For this review, take the finished solid that the model builds, in its own axes (mm). A direction names the side the tool comes from. Give positions to 0.01 mm unless a question says otherwise; leave off trailing zeros. Write each loop counter-clockwise with the first axis right and the second up, starting at its lowest first coordinate (ties: lowest second). Pieces come first, ordered by that corner, then holes.
1) For P1, Ø3, axis at x = 16, z = 97, coming from the +Y side; P2, Ø3, axis at x = -2.5, y = 36.5, coming from the +Z side; P3, Ø6, axis at y = 0, z = 87.04, coming from the +X side, all flat-tipped, find the tip position at first contact; note any pin that passes through.
2) Draft analysis for pull direction X (two halves, no side actions). For faces 1 (the face through (-0.488, -13.131, 84.473)), 2 (the face through (0, 10, 75)), 3 (the face through (28.61, 8.75, 96.29)), state which applies: pulls with the +X half, pulls with the -X half, needs draft (parallel to the pull), parting line crosses it, or undercut.
3) Wall thickness on line 1 along Y through (x, z) = (25, 95); line 2 along Y through (x, z) = (-4, 102); line 3 along Z through (x, y) = (-5.5, 33): over which ranges is each line inside the solid? List them lowest first.
4) We need section D-D on z = 88. Give the boundary of the cut face in (x, y).
5) Machinability: for faces 4 (the face through (5, 36, 78.039)), 5 (the face through (16.35, -1, 96)), 6 (the face through (37.42, 15.57, 74.82)), which of the approach directions +Z, -Z, +X, -X, +Y, -Y give a long, thin tool a straight path to every point of the face, cutting with its end or side? Answer none if there is none.
6) We need section C-C on x = 31. Give the boundary of the cut face in (y, z).
7) We need section A-A on x = 0. Give the boundary of the cut face in (y, z), and give its area (3 significant figures).
8) We need section B-B on y = 0. Give the boundary of the cut face in (x, z), and give its area (3 significant figures).
from build123d import *

# Parameters (mm, degrees)
SKETCH2_W            = 6.35
SKETCH2_H            = 20
BOSS_EXTRUDE1_DEPTH  = 42.349999882
SKETCH3_R            = 1.7
SKETCH3_W            = 24.870089154
SKETCH3_H            = 26.35
SKETCH3_W_2          = 9.220089154
SKETCH3_H_2          = 42
BOSS_EXTRUDE2_DEPTH  = 6.35
BOSS_EXTRUDE4_DEPTH  = 6.35
M4_CLEARANCE_HOLE1_D = 4.5
M4_CLEARANCE_HOLE2_D = 4.5
BOSS_EXTRUDE5_DEPTH  = 2.54


with BuildPart() as part:
    # Sketch2 → Boss-Extrude1 (new body)
    with BuildSketch(Plane.XY.offset(114.038644373)):
        Polygon((16.35, -10), (10, -10), (-10, -10), (-10, -16.35), (16.35, -16.35), align=None)
        with Locations((13.175, 0)):
            Rectangle(SKETCH2_W, SKETCH2_H)
    extrude(amount=-BOSS_EXTRUDE1_DEPTH)

    # Sketch3 → Boss-Extrude2 (add)
    # profile 1 of 4: a face of its own
    with BuildSketch(Plane(origin=(0, 0, 71.688644491), x_dir=(-1, 0, 0), z_dir=(0, 0, -1))):
        with BuildLine():
            Line((-41.220089154, 10), (-16.35, 10))
            Line((-16.35, 10), (-16.35, 15.990922415))
            ThreePointArc((-16.35, 15.990922415), (-32.472362042, 40.493777386), (-4.720089154, 31))
            ThreePointArc((-4.720089154, 31), (-7.596369472, 22.006018601), (-15.157728044, 16.35))
            Line((-15.157728044, 16.35), (-6.19233234, 16.35))
            ThreePointArc((-6.19233234, 16.35), (-4.720089154, 17.2), (-3.247845967, 16.35))
            Line((-3.247845967, 16.35), (0.779910846, 16.35))
            Line((0.779910846, 16.35), (0.779910846, 52))
            Line((0.779910846, 52), (-41.220089154, 52))
            Line((-41.220089154, 52), (-41.220089154, 10))
        make_face()
        with Locations((-35.720089154, 15.5)):
            Circle(SKETCH3_R, mode=Mode.SUBTRACT)
        with Locations((-35.720089154, 46.5)):
            Circle(SKETCH3_R, mode=Mode.SUBTRACT)
        with Locations((-4.720089154, 46.5)):
            Circle(SKETCH3_R, mode=Mode.SUBTRACT)
    # profile 2 of 4: a face of its own
    with BuildSketch(Plane(origin=(0, 0, 71.688644491), x_dir=(-1, 0, 0), z_dir=(0, 0, -1))):
        with Locations((-28.785044577, -3.175)):
            Rectangle(SKETCH3_W, SKETCH3_H)
    # profile 3 of 4: a face of its own
    with BuildSketch(Plane(origin=(0, 0, 71.688644491), x_dir=(-1, 0, 0), z_dir=(0, 0, -1))):
        with BuildLine():
            Line((-16.35, 15.990922415), (-16.35, 10))
            Line((-16.35, 10), (-10, 10))
            Line((-10, 10), (0.779910846, 10))
            Line((0.779910846, 10), (0.779910846, 16.35))
            Line((0.779910846, 16.35), (-3.247845967, 16.35))
            ThreePointArc((-3.247845967, 16.35), (-3.078015249, 15.939992377), (-3.020089154, 15.5))
            ThreePointArc((-3.020089154, 15.5), (-5.16008153, 13.857926095), (-6.19233234, 16.35))
            Line((-6.19233234, 16.35), (-15.157728044, 16.35))
            ThreePointArc((-15.157728044, 16.35), (-15.750256819, 16.158483942), (-16.35, 15.990922415))
        make_face()
    # profile 4 of 4: a face of its own
    with BuildSketch(Plane(origin=(0, 0, 71.688644491), x_dir=(-1, 0, 0), z_dir=(0, 0, -1))):
        with Locations((5.389955423, 31)):
            Rectangle(SKETCH3_W_2, SKETCH3_H_2)
    extrude(amount=-BOSS_EXTRUDE2_DEPTH)

    # Sketch4 → Boss-Extrude4 (add)
    with BuildSketch(Plane.XZ.offset(16.35)):
        Polygon((16.35, 114.038644373), (41.220089154, 78.038644491), (16.35, 78.038644491), align=None)
    extrude(amount=-BOSS_EXTRUDE4_DEPTH)

    # M4 Clearance Hole1 (through all)
    with Locations(Plane(origin=(16.35, 0, 0), x_dir=(0, 0, -1), z_dir=(1, 0, 0))):
        with Locations((-105.038644403, 0), (-87.038644462, 0)):
            Hole(M4_CLEARANCE_HOLE1_D / 2)

    # M4 Clearance Hole2 (through all)
    with Locations(Plane(origin=(0, -16.35, 0), x_dir=(-1, 0, 0), z_dir=(0, -1, 0))):
        with Locations((0, -82.276144462), (0, -103.451144403)):
            Hole(M4_CLEARANCE_HOLE2_D / 2)

    # Sketch11 → Boss-Extrude5 (add)
    with BuildSketch(Plane(origin=(0, 10, 0), x_dir=(1, 0, 0), z_dir=(0, 1, 0))):
        Polygon((16.35, -114.038644373), (41.220089154, -78.038644491), (16.35, -78.038644491), align=None)
    extrude(amount=-BOSS_EXTRUDE5_DEPTH)


solid = part.part
Results list:
1. P1: stops at y = 10
1. P2: stops at z = 78.04
1. P3: stops at x = 16.35
2. face 1: undercut
2. face 2: needs draft
2. face 3: pulls with the +X half
3. line 1: y = -16.35 to -10, 7.46 to 10
3. line 2: y = -16.35 to -10
3. line 3: z = 71.69 to 78.04
4. outline: (-10, -16.35) - (34.34, -16.35) - (34.34, -10) - (16.35, -10) - (16.35, -2.03) - (10, -2.03) - (10, -10) - (-10, -10) - close; (10, 2.03) - (16.35, 2.03) - (16.35, 7.46) - (34.34, 7.46) - (34.34, 10) - (10, 10) - close
5. face 4: +Z, +X, -X, +Y
5. face 5: +Z, +X
5. face 6: +Z, -Z
6. outline: (-16.35, 71.69) - (19.86, 71.69) - (19.86, 78.04) - (10, 78.04) - (10, 92.83) - (7.46, 92.83) - (7.46, 78.04) - (-10, 78.04) - (-10, 92.83) - (-16.35, 92.83) - close; (42.14, 71.69) - (52, 71.69) - (52, 78.04) - (42.14, 78.04) - close
7. outline: (-16.35, 71.69) - (-10, 71.69) - (-10, 80.03) - (-16.35, 80.03) - close; (-16.35, 84.53) - (-10, 84.53) - (-10, 101.2) - (-16.35, 101.2) - close; (-16.35, 105.7) - (-10, 105.7) - (-10, 114.04) - (-16.35, 114.04) - close; (10, 71.69) - (52, 71.69) - (52, 78.04) - (10, 78.04) - close
7. area: 478 mm2
8. outline: (10, 71.69) - (41.22, 71.69) - (41.22, 78.04) - (16.35, 78.04) - (16.35, 84.79) - (10, 84.79) - close; (10, 89.29) - (16.35, 89.29) - (16.35, 102.79) - (10, 102.79) - close; (10, 107.29) - (16.35, 107.29) - (16.35, 114.04) - (10, 114.04) - close
8. area: 370 mm2
